The model under review builds one solid part; all positions refer to its coordinate system, in mm. Round coordinates to 2 decimals unless told otherwise and drop trailing zeros. Order: outer loops, then holes, each group sorted by start corner. A loop starts at its lowest first (then second) coordinate and runs counter-clockwise, first axis right, second up.
1) To check wall thickness, follow L1, parallel to Z at x = -2, y = 2.1; L2, parallel to Y at x = -6, z = -6; L3, parallel to X at y = 2.15, z = 9.5. State the ranges of each line that lie inside material, in increasing order.
2) Mouldability with a two-part tool opening along X and no side actions: class faces 1 (the face through (-2, 2, 0)), 2 (the face through (4.336, 1.282, 19.524)), 3 (the face through (1, 2.6, 0)) as pulls with the +X half, pulls with the -X half, needs draft (parallel to the pull), parting line crosses it, or undercut.
3) Consider section B-B (x = 10.5). Give the boundary of the cut face in (y, z).
4) Clearance check with flat-ended pins moving along their axes: P1, Ø12, axis at x = 13.5, z = 13, coming from the -Y side; P2, Ø0.7, axis at x = -1.5, y = 2.5, coming from the -Z side; P3, Ø0.7, axis at y = 2, z = -6.5, coming from the -X side; P4, Ø0.5, axis at x = -1.5, y = 2, coming from the +Z side. State where each tip first meets the part, or that it passes through.
5) Consider section A-A (y = 0.8). Give the boundary of the cut face in (x, z), then the cut area to 3 significant figures.
Autodesk Inventor part; units mm, degrees
ref_plane "YZ Plane" through (0, 0, 0) normal (1, 0, 0) x (0, 1, 0)
ref_plane "XZ Plane" through (0, 0, 0) normal (0, 1, 0) x (-1, 0, 0)
ref_plane "XY Plane" through (0, 0, 0) normal (0, 0, 1) x (1, 0, 0)
sketch "Sketch1" plane through (0, 0, 0) normal (0, 1, 0) x (-1, 0, 0)
  circle A0 centre (0, 0) radius 20
  dimension "d0" = 40
extrude "Extrusion1" add sketch "Sketch1" along normal blind 2.6
sketch "Sketch2" plane through (0, 2.6, 0) normal (0, 1, 0) x (1, 0, 0)
  line L0 (-10, -10) -> (-10, 10)
  line L1 (-10, 10) -> (10, 10)
  line L2 (10, 10) -> (10, -10)
  line L3 (10, -10) -> (-10, -10)
  line L4 (-10, -10) -> (10, 10) construction
  line L5 (-10, 10) -> (10, -10) construction
  point P0 (0, 0)
  dimension "d3" = 20
  dimension "d4" = 20
extrude "Extrusion2" cut sketch "Sketch2" against normal blind 0.6
sketch "Sketch3" plane through (0, 2, 0) normal (0, 1, 0) x (1, 0, 0)
  line L0 (-6.2284, 8.788) -> (6.2284, 8.788) construction
  line L1 (6.2284, 8.788) -> (6.2284, -8.5115) construction
  line L2 (6.2284, -8.5115) -> (-6.2284, -8.5115) construction
  line L3 (-6.2284, -8.5115) -> (-6.2284, 8.788) construction
  spline S0 degree 2 poles (-0.5381, 6.8643) (-1.1434, 6.8643) (-2.3407, 6.5684) (-2.9191, 6.3397) knots 0 0 0 1 2 2 2
  spline S1 degree 2 poles (-2.9191, 6.3397) (-3.4572, 6.111) (-4.2509, 5.6267) (-4.5603, 5.4115) knots 0 0 0 1 2 2 2
  line L4 (-4.5603, 5.4115) -> (-4.6948, 5.4115)
  line L5 (-4.6948, 5.4115) -> (-4.6948, 7.7656)
  spline S2 degree 2 poles (-4.6948, 7.7656) (-3.9684, 8.1557) (-1.4797, 8.788) (-0.3632, 8.788) knots 0 0 0 1 2 2 2
  spline S3 degree 2 poles (-0.3632, 8.788) (0.7668, 8.788) (2.4483, 8.3306) (3.1344, 7.8463) knots 0 0 0 1 2 2 2
  spline S4 degree 2 poles (3.1344, 7.8463) (3.8608, 7.3217) (4.6141, 5.8016) (4.6141, 4.7792) knots 0 0 0 1 2 2 2
  spline S5 degree 2 poles (4.6141, 4.7792) (4.6141, 3.4071) (2.8115, 1.3355) (1.547, 1.0664) knots 0 0 0 1 2 2 2
  line L6 (1.547, 1.0664) -> (1.547, 0.905)
  spline S6 degree 2 poles (1.547, 0.905) (2.0716, 0.7974) (3.2689, 0.3131) (3.7801, -0.1712) knots 0 0 0 1 2 2 2
  spline S7 degree 2 poles (3.7801, -0.1712) (4.2912, -0.642) (4.937, -2.1487) (4.937, -3.2383) knots 0 0 0 1 2 2 2
  spline S8 degree 2 poles (4.937, -3.2383) (4.937, -4.3548) (4.1702, -6.2516) (3.4707, -6.978) knots 0 0 0 1 2 2 2
  spline S9 degree 2 poles (3.4707, -6.978) (2.7442, -7.7313) (0.6861, -8.5115) (-0.6188, -8.5115) knots 0 0 0 1 2 2 2
  spline S10 degree 2 poles (-0.6188, -8.5115) (-1.8699, -8.5115) (-4.3182, -7.9062) (-5.1522, -7.4892) knots 0 0 0 1 2 2 2
  line L7 (-5.1522, -7.4892) -> (-5.1522, -5.135)
  line L8 (-5.1522, -5.135) -> (-4.9908, -5.135)
  spline S11 degree 2 poles (-4.9908, -5.135) (-4.2912, -5.6462) (-1.9237, -6.5879) (-0.7533, -6.5879) knots 0 0 0 1 2 2 2
  spline S12 degree 2 poles (-0.7533, -6.5879) (-0.0673, -6.5879) (1.3049, -6.1574) (1.7622, -5.6597) knots 0 0 0 1 2 2 2
  spline S13 degree 2 poles (1.7622, -5.6597) (2.2062, -5.162) (2.677, -3.9782) (2.677, -3.0769) knots 0 0 0 1 2 2 2
  spline S14 degree 2 poles (2.677, -3.0769) (2.677, -2.1756) (2.1524, -1.0052) (1.6815, -0.6689) knots 0 0 0 1 2 2 2
  spline S15 degree 2 poles (1.6815, -0.6689) (1.2107, -0.3326) (-0.0673, -0.077) (-0.8206, -0.077) knots 0 0 0 1 2 2 2
  line L9 (-0.8206, -0.077) -> (-1.7622, -0.077)
  line L10 (-1.7622, -0.077) -> (-1.7622, 1.7659)
  line L11 (-1.7622, 1.7659) -> (-1.0224, 1.7659)
  spline S16 degree 2 poles (-1.0224, 1.7659) (0.4708, 1.7659) (2.3541, 3.1919) (2.3541, 4.5505) knots 0 0 0 1 2 2 2
  spline S17 degree 2 poles (2.3541, 4.5505) (2.3541, 5.1828) (1.8699, 6.0841) (1.4797, 6.3531) knots 0 0 0 1 2 2 2
  spline S18 degree 2 poles (1.4797, 6.3531) (1.0627, 6.6356) (0.0404, 6.8643) (-0.5381, 6.8643) knots 0 0 0 1 2 2 2
  point P0 (0, 0)
extrude "Extrusion3" add sketch "Sketch3" along normal blind 0.6
properties part number "TopMarker3"
Answer below:
1. L1: z = -19.9 to -10, -8.63 to -6.65, 6.46 to 8.42, 10 to 19.9
1. L2: y = 0 to 2
1. L3: x = -17.6 to -10, 10 to 17.6
2. face 1: undercut
2. face 2: parting line crosses it
2. face 3: needs draft
3. outline: (0, -17.02) - (2.6, -17.02) - (2.6, 17.02) - (0, 17.02) - close
4. P1: stops at y = 0
4. P2: stops at z = -19.97
4. P3: stops at x = -19.03
4. P4: stops at z = 19.96
5. outline: circle Ø40 at (0, 0)
5. area: 1,260 mm2
